Can you work these out from the model? Positions are in its coordinate system, mm. A direction names the side the tool comes from. Give positions to 0.01 mm unless a question says otherwise; leave off trailing zeros. Loops run counter-clockwise (first coordinate to the right, second up) from the corner with the lowest first, then second, coordinate; pieces in that order, holes last.
from build123d import *

# Parameters (mm, degrees)
SKETCH_1_W           = 30
SKETCH_1_H           = 59.5
EXTRUDE_1_DEPTH      = 1.5
SKETCH_2_W           = 20
SKETCH_2_H           = 55
CUT_EXTRUDE_1_DEPTH  = 0.1
SKETCH_3_R           = 5
EXTRUDE_2_DEPTH      = 0.1
EXTRUDE_3_DEPTH      = 0.1
CUT_EXTRUDE_START    = -0.1
SKETCH_5_R           = 5
CUT_EXTRUDE_2_DEPTH  = 0.1
SKETCH_6_R           = 3
CUT_EXTRUDE_3_DEPTH  = 0.1
CUT_EXTRUDE_4_DEPTH  = 0.1
SKETCH_8_R           = 3
CUT_EXTRUDE_5_DEPTH  = 0.1
SKETCH_9_W           = 1
SKETCH_9_H           = 10
CUT_EXTRUDE_6_DEPTH  = 0.1
SKETCH_10_R          = 0.25
EXTRUDE_4_DEPTH      = 0.1
SKETCH_11_W          = 2
SKETCH_11_H          = 12
EXTRUDE_5_DEPTH      = 1.5
CUT_EXTRUDE_7_DEPTH  = 42.654081433
SKETCH_13_W          = 2
SKETCH_13_H          = 12
EXTRUDE_6_DEPTH      = 2
CUT_EXTRUDE_8_DEPTH  = 42.654081433
CUT_EXTRUDE_9_DEPTH  = 42.654081433
CUT_EXTRUDE_10_DEPTH = 42.654081433
SKETCH_18_R          = 0.5
EXTRUDE_7_DEPTH      = 59.5
SKETCH_19_W          = 1
SKETCH_19_H          = 56.9
CUT_EXTRUDE_11_DEPTH = 2


with BuildPart() as part:
    # 草圖1 → 填料-伸長1 (new body)
    with BuildSketch(Plane.XY):
        Rectangle(SKETCH_1_W, SKETCH_1_H)
    extrude(amount=EXTRUDE_1_DEPTH)

    # 草圖2 → 除料-伸長1 (cut)
    with BuildSketch(Plane.XY.offset(1.5)):
        Rectangle(SKETCH_2_W, SKETCH_2_H)
    extrude(amount=-CUT_EXTRUDE_1_DEPTH, mode=Mode.SUBTRACT)

    # 草圖3 → 填料-伸長2 (add)
    with BuildSketch(Plane.XY.offset(1.4)):
        Circle(SKETCH_3_R)
    extrude(amount=EXTRUDE_2_DEPTH)

    # 草圖4 → 填料-伸長3 (add)
    with BuildSketch(Plane.XY.offset(1.4)):
        with BuildLine():
            ThreePointArc((4.993746089, 0.25), (7.506502742, 0.566687178), (10, 1.010205144))
            Line((10, 1.010205144), (10, 27.5))
            Line((10, 27.5), (8.241767279, 27.5))
            ThreePointArc((8.241767279, 27.5), (2.882359671, 16.731048078), (0.25, 4.993746089))
            ThreePointArc((0.25, 4.993746089), (3.535533906, 3.535533906), (4.993746089, 0.25))
        make_face()
        with BuildLine():
            ThreePointArc((0.25, -4.993746089), (2.882359671, -16.731048078), (8.241767279, -27.5))
            Line((8.241767279, -27.5), (10, -27.5))
            Line((10, -27.5), (10, -1.010205144))
            ThreePointArc((10, -1.010205144), (7.506502742, -0.566687178), (4.993746089, -0.25))
            ThreePointArc((4.993746089, -0.25), (3.535533906, -3.535533906), (0.25, -4.993746089))
        make_face()
        with BuildLine():
            Line((-10, -27.5), (-8.241767279, -27.5))
            ThreePointArc((-8.241767279, -27.5), (-2.882359671, -16.731048078), (-0.25, -4.993746089))
            ThreePointArc((-0.25, -4.993746089), (-3.535533906, -3.535533906), (-4.993746089, -0.25))
            ThreePointArc((-4.993746089, -0.25), (-7.506502742, -0.566687178), (-10, -1.010205144))
            Line((-10, -1.010205144), (-10, -27.5))
        make_face()
        with BuildLine():
            Line((-10, 27.5), (-10, 1.010205144))
            ThreePointArc((-10, 1.010205144), (-7.506502742, 0.566687178), (-4.993746089, 0.25))
            ThreePointArc((-4.993746089, 0.25), (-3.535533906, 3.535533906), (-0.25, 4.993746089))
            ThreePointArc((-0.25, 4.993746089), (-2.882359671, 16.731048078), (-8.241767279, 27.5))
            Line((-8.241767279, 27.5), (-10, 27.5))
        make_face()
    extrude(amount=EXTRUDE_3_DEPTH)

    # 草圖5 → 除料-伸長2 (cut)
    with BuildSketch(Plane.XY.offset(1.5).offset(CUT_EXTRUDE_START)):
        Circle(SKETCH_5_R)
    extrude(amount=CUT_EXTRUDE_2_DEPTH, mode=Mode.SUBTRACT)

    # 草圖6 → 除料-伸長3 (cut)
    with BuildSketch(Plane.XY.offset(1.4)):
        Circle(SKETCH_6_R)
    extrude(amount=-CUT_EXTRUDE_3_DEPTH, mode=Mode.SUBTRACT)

    # 草圖7 → 除料-伸長4 (cut)
    with BuildSketch(Plane(origin=(0, 0, 0), x_dir=(-1, 0, 0), z_dir=(0, 0, -1))):
        with BuildLine():
            Line((-8.241767279, -27.5), (8.241767279, -27.5))
            ThreePointArc((8.241767279, -27.5), (2.882359671, -16.731048078), (0.25, -4.993746089))
            ThreePointArc((0.25, -4.993746089), (3.535533906, -3.535533906), (4.993746089, -0.25))
            ThreePointArc((4.993746089, -0.25), (7.506502742, -0.566687178), (10, -1.010205144))
            Line((10, -1.010205144), (10, 1.010205144))
            ThreePointArc((10, 1.010205144), (7.506502742, 0.566687178), (4.993746089, 0.25))
            ThreePointArc((4.993746089, 0.25), (3.535533906, 3.535533906), (0.25, 4.993746089))
            ThreePointArc((0.25, 4.993746089), (2.882359671, 16.731048078), (8.241767279, 27.5))
            Line((8.241767279, 27.5), (-8.241767279, 27.5))
            ThreePointArc((-8.241767279, 27.5), (-2.882359671, 16.731048078), (-0.25, 4.993746089))
            ThreePointArc((-0.25, 4.993746089), (-3.535533906, 3.535533906), (-4.993746089, 0.25))
            ThreePointArc((-4.993746089, 0.25), (-7.506502742, 0.566687178), (-10, 1.010205144))
            Line((-10, 1.010205144), (-10, -1.010205144))
            ThreePointArc((-10, -1.010205144), (-7.506502742, -0.566687178), (-4.993746089, -0.25))
            ThreePointArc((-4.993746089, -0.25), (-3.535533906, -3.535533906), (-0.25, -4.993746089))
            ThreePointArc((-0.25, -4.993746089), (-2.882359671, -16.731048078), (-8.241767279, -27.5))
        make_face()
    extrude(amount=-CUT_EXTRUDE_4_DEPTH, mode=Mode.SUBTRACT)

    # 草圖8 → 除料-伸長5 (cut)
    with BuildSketch(Plane(origin=(0, 0, 0.1), x_dir=(-1, 0, 0), z_dir=(0, 0, -1)).offset(CUT_EXTRUDE_START)):
        with Locations(Location((0, 0, 0), (0, 0, 180))):
            Circle(SKETCH_8_R)
    extrude(amount=CUT_EXTRUDE_5_DEPTH, mode=Mode.SUBTRACT)

    # 草圖9 → 除料-伸長6 (cut)
    with BuildSketch(Plane(origin=(15, 0, 0), x_dir=(0, 0, -1), z_dir=(1, 0, 0))):
        with Locations((-0.75, 0)):
            Rectangle(SKETCH_9_W, SKETCH_9_H)
    extrude(amount=-CUT_EXTRUDE_6_DEPTH, mode=Mode.SUBTRACT)

    # 草圖10 → 填料-伸長4 (add)
    with BuildSketch(Plane(origin=(14.9, 0, 0), x_dir=(0, 0, -1), z_dir=(1, 0, 0))):
        with Locations((-0.75, -3)):
            Circle(SKETCH_10_R)
        with Locations((-0.75, -1.7)):
            Circle(SKETCH_10_R)
        with Locations((-0.75, -0.4)):
            Circle(SKETCH_10_R)
        with Locations((-0.75, 0.9)):
            Circle(SKETCH_10_R)
        with Locations((-0.75, 2.2)):
            Circle(SKETCH_10_R)
    extrude(amount=EXTRUDE_4_DEPTH)

    # 草圖11 → 填料-伸長5 (add)
    with BuildSketch(Plane.XY.offset(1.5)):
        with Locations((13, 0)):
            Rectangle(SKETCH_11_W, SKETCH_11_H)
    extrude(amount=EXTRUDE_5_DEPTH)

    # 草圖12 → 除料-伸長7 (cut, through all)
    with BuildSketch(Plane(origin=(14, 0, 0), x_dir=(0, 0, -1), z_dir=(1, 0, 0))):
        Polygon((-1.8, 6), (-1.8, -3.892813963), (-2.45595706, -3.892813963), (-2.301062562, -0.267088334), (-2.736577143, -0.267088334), (-3, -3.073435974), (-3, 6), align=None)
        Polygon((-3, -6), (-1.8, -6), (-1.8, -5.188306953), (-2.363031893, -5.188306953), (-2.363031893, -5.650911739), (-2.678275837, -5.650911739), (-3, -4.356848884), align=None)
    extrude(amount=-CUT_EXTRUDE_7_DEPTH, mode=Mode.SUBTRACT)

    # 草圖13 → 填料-伸長6 (add)
    with BuildSketch(Plane(origin=(0, 0, 0), x_dir=(-1, 0, 0), z_dir=(0, 0, -1))):
        with Locations((-13, 0)):
            Rectangle(SKETCH_13_W, SKETCH_13_H)
    extrude(amount=EXTRUDE_6_DEPTH)

    # 草圖14 → 除料-伸長8 (cut, through all)
    with BuildSketch(Plane(origin=(14, 0, 0), x_dir=(0, 0, -1), z_dir=(1, 0, 0))):
        Polygon((1.152930519, 6), (2, -2.477443224), (2, 6), align=None)
        Polygon((2, -4.322370965), (1.57646526, -6), (2, -6), align=None)
    extrude(amount=-CUT_EXTRUDE_8_DEPTH, mode=Mode.SUBTRACT)

    # 草圖15 → 除料-伸長9 (cut, through all)
    with BuildSketch(Plane(origin=(14, 0, 0), x_dir=(0, 0, -1), z_dir=(1, 0, 0))):
        Polygon((0.753392093, 6), (1.537923786, -1.851567128), (1.145657939, -1.979765392), (0.570903406, 3.772358885), (0, 3.772358885), (0, 6), align=None)
    extrude(amount=-CUT_EXTRUDE_9_DEPTH, mode=Mode.SUBTRACT)

    # 草圖17 → 除料-伸長10 (cut, through all)
    with BuildSketch(Plane(origin=(14, 0, 0), x_dir=(0, 0, -1), z_dir=(1, 0, 0))):
        Polygon((0.570903406, 3.772358885), (0.570903406, -1.986165117), (1.145657939, -1.979765392), align=None)
    extrude(amount=-CUT_EXTRUDE_10_DEPTH, mode=Mode.SUBTRACT)

    # 草圖18 → 填料-伸長7 (add, through all)
    with BuildSketch(Plane(origin=(0, 29.75, 0), x_dir=(1, 0, 0), z_dir=(0, 1, 0))):
        with Locations((-14.5, -2)):
            Circle(SKETCH_18_R)
        with BuildLine():
            Line((-14.5, -1.5), (-15, -1.5))
            Line((-15, -1.5), (-15, -2))
            ThreePointArc((-15, -2), (-14.853553391, -1.646446609), (-14.5, -1.5))
        make_face()
    extrude(amount=-EXTRUDE_7_DEPTH)

    # 草圖19 → 除料-伸長11 (cut)
    with BuildSketch(Plane.ZY.offset(15)):
        with Locations((2, 0)):
            Rectangle(SKETCH_19_W, SKETCH_19_H)
    extrude(amount=-CUT_EXTRUDE_11_DEPTH, mode=Mode.SUBTRACT)


solid = part.part
(1) Suppose I cut it at B-B on x = -9.25. List the corners of the cut face in (y, z) for me, plus the area to 3 significant figures.
Returned:
outline: (-29.75, 0) - (-0.86, 0) - (-0.86, 0.1) - (0.86, 0.1) - (0.86, 0) - (29.75, 0) - (29.75, 1.5) - (0.86, 1.5) - (0.86, 1.4) - (-0.86, 1.4) - (-0.86, 1.5) - (-29.75, 1.5) - close
area: 88.9 mm2
(2) Suppose I cut it at A-A on y = 17. List the corners of the cut face in (x, z) for me, plus the area to 3 significant figures.
Returned:
outline: (-15, 0) - (-2.98, 0) - (-2.98, 0.1) - (2.98, 0.1) - (2.98, 0) - (15, 0) - (15, 1.5) - (2.98, 1.5) - (2.98, 1.4) - (-2.98, 1.4) - (-2.98, 1.5) - (-15, 1.5) - close
area: 43.8 mm2
(3) Thinking about a two-plate mould opening in X: for faces 1 (the flat face through (15, -7, 1)), 2 (the flat face through (13.01, 2.13, -1.14)), 3 (the flat face through (0, 0, 0.2)), which applies, pulls with the +X half, pulls with the -X half, needs draft (parallel to the pull), parting line crosses it, or undercut?
Returned:
face 1: pulls with the +X half
face 2: needs draft
face 3: undercut
(4) Which directions (+Z, -Z, +X, -X, +Y, -Y) give clear straight access to the entire face, cutting with the end or side of a thin tool? Please do faces 4 (the flat face through (13, -6, -1)), 5 (the flat face through (13.014, -1.651, 2.866)), 6 (the flat face through (13, 1, -0.571)).
Returned:
face 4: -Z, +X, -X, -Y
face 5: +Z, +X, -X, +Y
face 6: +X, -X, +Y
(5) Please list where these lines run through material, in increasing order: probe 1 along Y at (x, z) = (0, 1.35); probe 2 along X at (y, z) = (0, 1.45); probe 3 along Z at (x, y) = (-10.5, -17).
Returned:
probe 1: y = -29.75 to -3, 3 to 29.75
probe 2: x = -15 to -10, 10 to 15
probe 3: z = 0 to 1.5
(6) Will these pins go through, and if not, where does the flat tip stop? P1, Ø12, axis at x = -1.5, y = 6.5, coming from the +Z side; P2, Ø15, axis at x = -1.5, y = 5, coming from the -Z side; P3, Ø3.5, axis at x = 0, y = 0, coming from the -Z side.
Returned:
P1: stops at z = 1.5
P2: stops at z = 0
P3: stops at z = 0.2
